from build123d import *

# Parameters (mm, degrees)
EXTRUDE_1_DEPTH     = 10
SKETCH_2_OUTSIDE_W  = 16.288
SKETCH_2_OUTSIDE_H  = 20.288
SKETCH_2_OUTSIDE_R  = 2
CUT_EXTRUDE_3_DEPTH = 20.324595727


with BuildPart() as part:
    # Эскиз1 → Бобышка-Вытянуть1 (new body)
    with BuildSketch(Plane.XY):
        Polygon((-6.4, 0), (6.4, 0), (6.4, 2.5), (2.4, 2.5), (2.4, 14), (-2.4, 14), (-2.4, 2.5), (-6.4, 2.5), align=None)
    extrude(amount=EXTRUDE_1_DEPTH)

    # Эскиз2 outside → Вырез-Вытянуть3 (cut, through all)
    # profile 1 of 2: a face of its own
    with BuildSketch(Plane(origin=(2.4, 0, 0), x_dir=(0, 0, -1), z_dir=(1, 0, 0))):
        with Locations((-5, 7)):
            Rectangle(SKETCH_2_OUTSIDE_W, SKETCH_2_OUTSIDE_H)
        with BuildLine():
            Line((-10, 9), (-10, 0))
            Line((-10, 0), (0, 0))
            Line((0, 0), (0, 9))
            ThreePointArc((0, 9), (-5, 14), (-10, 9))
        make_face(mode=Mode.SUBTRACT)
    # profile 2 of 2: a face of its own
    with BuildSketch(Plane(origin=(2.4, 0, 0), x_dir=(0, 0, -1), z_dir=(1, 0, 0))):
        with Locations(Location((-5, 9, 0), (0, 0, 90))):
            Circle(SKETCH_2_OUTSIDE_R)
    extrude(amount=-CUT_EXTRUDE_3_DEPTH, mode=Mode.SUBTRACT)


solid = part.part
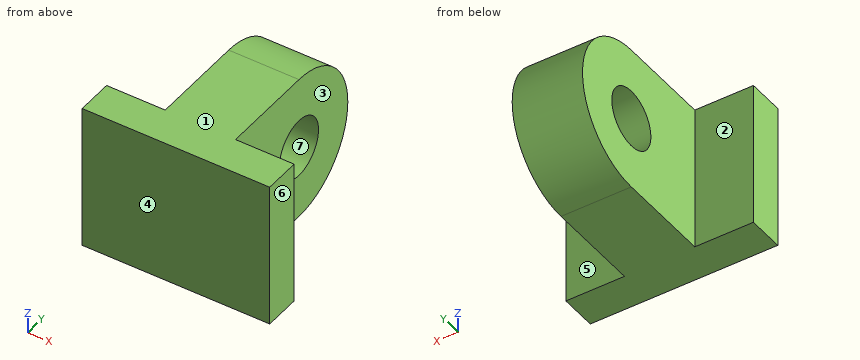
Model file for the job. Use its own axes, mm. Face numbers are marked on the shaded views. A direction names the side the tool comes from. Coordinates: 2 decimals unless noted, no trailing zeros. Loops run counter-clockwise (first coordinate to the right, second up) from the corner with the lowest first, then second, coordinate; pieces in that order, holes last. Notation, with made-up numbers: (-22, -11) -> (0, -11) arc R23 ccw to (0, 0) -> close; hole circle Ø5 at (2.5, -33). An arc over 180 degrees is marked (long way). Use one line per item in the form item = value. Start each with the question number.
(1) Cut at A-A on z = 5. Give the cut face in (x, y).
(2) Probe probe 1 along Z at (x, y) = (-0.1, 9); probe 2 along X at (y, z) = (12, 7.5); probe 3 along Y at (x, z) = (-3.75, 3). List the from-to ranges inside material, lowest first. Write a range as from..to.
(3) Flat gauge pins, fed straight in: pin 1 (4.5 mm diameter, centred on x = 3.5, z = 6, fed in from +Y); pin 2 (2 mm diameter, centred on x = -4, z = 5.5, fed in from +Y); pin 3 (4.5 mm diameter, centred on y = 9, z = 5, fed in from -X). Where does each tip first touch, or does it go through?
(4) Tool access for the marked faces 1, 2 and 3: list every direction of +Z, -Z, +X, -X, +Y, -Y with a clear straight run to the whole face (end or side of a thin tool).
(5) Pull direction Y, two halves, no side cores. Call the marked faces 4, 5, 6 and 7: pulls with the +Y half, pulls with the -Y half, needs draft (parallel to the pull), parting line crosses it, or undercut.
(6) Cut at B-B on x = 2. Give the cut face in (y, z).
(7) Cut at D-D on x = 5.75. Give the cut face in (y, z), and give its area (3 significant figures).
(8) Cut at C-C on z = 8. Give the cut face in (x, y), and give its area (3 significant figures).
Values:
q1.outline = (-6.4, 0) -> (6.4, 0) -> (6.4, 2.5) -> (2.4, 2.5) -> (2.4, 7) -> (-2.4, 7) -> (-2.4, 2.5) -> (-6.4, 2.5) -> close; (-2.4, 11) -> (2.4, 11) -> (2.4, 14) -> (-2.4, 14) -> close
q2.probe_1 = 0..3, 7..10
q2.probe_2 = -2.4..2.4
q2.probe_3 = 0..2.5
q3.pin_1 = 14
q3.pin_2 = 2.5
q3.pin_3 = -2.4
q4.face_1 = +Z, +X, -X, +Y, -Y
q4.face_2 = +Z, -Z, -X, +Y
q4.face_3 = +Z, -Z, +X, +Y
q5.face_4 = pulls with the -Y half
q5.face_5 = pulls with the +Y half
q5.face_6 = needs draft
q5.face_7 = undercut
q6.outline = (0, 0) -> (9, 0) arc R5 ccw to (9, 10) -> (0, 10) -> close; hole circle Ø4 at (9, 5)
q7.outline = (0, 0) -> (2.5, 0) -> (2.5, 10) -> (0, 10) -> close
q7.area = 25.0 mm2
q8.outline = (-6.4, 0) -> (6.4, 0) -> (6.4, 2.5) -> (2.4, 2.5) -> (2.4, 13) -> (-2.4, 13) -> (-2.4, 2.5) -> (-6.4, 2.5) -> close
q8.area = 82.4 mm2
